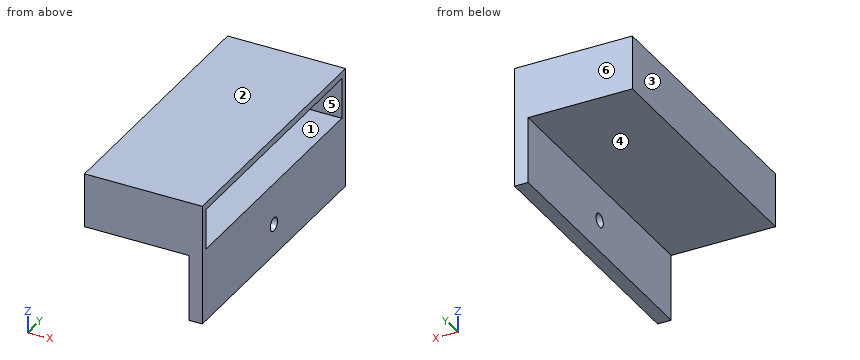
```python
from build123d import *

# Parameters (mm, degrees)
F0_W     = 3
F0_H     = 14.70934
F1_DEPTH = 59
F2_R     = 1.5
F3_DEPTH = 4
F2_W     = 56
F2_H     = 9
F4_DEPTH = 24


with BuildPart() as f1:
    # F0 (on Front) → F1 (new body)
    with BuildSketch(Plane.XZ):
        Polygon((-12, 12), (-38, 12), (-38, 0), (-15, 0), (-12, 0), align=None)
        with Locations((-13.5, -7.35467)):
            Rectangle(F0_W, F0_H)
    extrude(amount=F1_DEPTH)

    # F2 (on face) → F3 (cut)
    with BuildSketch(Plane.YZ.offset(-12)):
        with Locations((-29.5, -7.70934)):
            Circle(F2_R)
    extrude(amount=-F3_DEPTH, mode=Mode.SUBTRACT)

    # F2 (on face) → F4 (cut)
    with BuildSketch(Plane.YZ.offset(-12)):
        with Locations((-29.5, 6)):
            Rectangle(F2_W, F2_H)
        with Locations((-29.5, -7.70934)):
            Circle(F2_R)
    extrude(amount=-F4_DEPTH, mode=Mode.SUBTRACT)


solid = f1.part
```
Here's how the part is built. I have some questions about the finished solid (model axes, mm). Face numbers are marked on the shaded views. A direction names the side the tool comes from. Coordinates: 2 decimals unless noted, no trailing zeros. Write each loop counter-clockwise with the first axis right and the second up, starting at its lowest first coordinate (ties: lowest second). Pieces come first, ordered by that corner, then holes. Notation, with made-up numbers: M 11,22 L 17,22 A28 ccw 17,48 Z; hole C -26.75,31.5 d10. An arc over 180 degrees is marked long. Answer as CSV lines item,"result". Start each with the question number.
Q1. Suppose I cut it at C-C, the plane z = -1.5. List the corners of the cut face in (x, y) for me, then the cut area to 3 significant figures.
Q2. I need wall thicknesses on probe 1 along Z at (x, y) = (-14.1, -29.5); probe 2 along Z at (x, y) = (-30.25, -56); probe 3 along Y at (x, z) = (-27.75, 9.75). Which ranges of each line are inside material? Lowest first, please. Write a range as [from, to].
Q3. For the marked faces 4, 5 and 6, which set-ups out of +Z, -Z, +X, -X, +Y, -Y let a thin tool reach every point of the face, with its end or its side?
Q4. Will these pins go through, and if not, where does the flat tip stop? pin 1 Ø3 at (y, z) = (-29, 5) entering from +X; pin 2 Ø4 at (y, z) = (-12.5, -10) entering from -X; pin 3 Ø5 at (x, y) = (-32, -16) entering from -Z; pin 4 Ø3.5 at (y, z) = (-29.5, -7.71) entering from +X.
Q5. Suppose I cut it at B-B, the plane x = -16.5. List the corners of the cut face in (y, z) for me, then the cut area to 3 significant figures.
Q6. Suppose I cut it at A-A, the plane y = -29.5. List the corners of the cut face in (x, z) for me, then the cut area to 3 significant figures.
Q7. If we mould it in two halves opening along Z, with no side actions, what happens to the marked faces 1, 2 and 3? For each: pulls with the +Z half, pulls with the -Z half, needs draft (parallel to the pull), parting line crosses it, or undercut.
Entries:
1,outline,"M -15,-59 L -12,-59 L -12,0 L -15,0 Z"
1,area,"177 mm²"
2,probe 1,"z = [-14.71, -9.21], [-6.21, 1.5], [10.5, 12]"
2,probe 2,"z = [0, 1.5], [10.5, 12]"
2,probe 3,"y = [-59, -57.5], [-1.5, 0]"
3,face 4,"-Z, -X, +Y, -Y"
3,face 5,"+X"
3,face 6,"+Z, -Z, +X, -X, +Y"
4,pin 1,"stops at x = -36"
4,pin 2,"stops at x = -15"
4,pin 3,"stops at z = 0"
4,pin 4,"stops at x = -12"
5,outline,"M -59,0 L 0,0 L 0,12 L -59,12 Z; hole M -57.5,1.5 L -1.5,1.5 L -1.5,10.5 L -57.5,10.5 Z"
5,area,"204 mm²"
6,outline,"M -38,0 L -15,0 L -15,-6.21 L -12,-6.21 L -12,1.5 L -36,1.5 L -36,10.5 L -12,10.5 L -12,12 L -38,12 Z; M -15,-14.71 L -12,-14.71 L -12,-9.21 L -15,-9.21 Z"
6,area,"131 mm²"
7,face 1,"undercut"
7,face 2,"pulls with the +Z half"
7,face 3,"needs draft"
